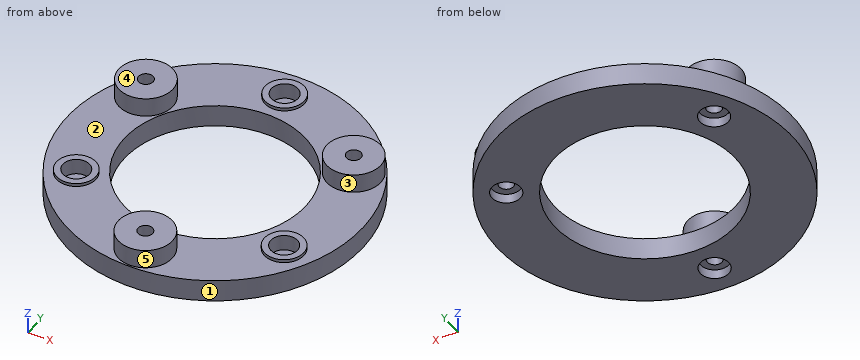
Autodesk Inventor part; units mm, degrees
ref_plane "YZ Plane" through (0, 0, 0) normal (1, 0, 0) x (0, 1, 0)
ref_plane "XZ Plane" through (0, 0, 0) normal (0, 1, 0) x (-1, 0, 0)
ref_plane "XY Plane" through (0, 0, 0) normal (0, 0, 1) x (1, 0, 0)
sketch "Skizze1" plane through (0, 0, 0) normal (0, 0, 1) x (1, 0, 0)
  line L0 (-32.55, 0) -> (32.55, 0) construction
  circle A0 centre (0, 0) radius 18.75 construction
  circle A1 centre (0, 18.75) radius 2.1
  circle A2 centre (16.238, -9.375) radius 2.1
  circle A3 centre (-16.238, -9.375) radius 2.1
  line L1 (0, 32.55) -> (0, -32.55) construction
  line L2 (0, 0) -> (-16.238, -9.375) construction
  circle A4 centre (0, 0) radius 14.25
  circle A5 centre (0, 0) radius 23.25
  circle A6 centre (0, -18.75) radius 1.15
  circle A7 centre (16.238, 9.375) radius 1.15
  circle A8 centre (-16.238, 9.375) radius 1.15
  circle A9 centre (0, -18.75) radius 4.25
  circle A10 centre (-16.238, 9.375) radius 4.25
  circle A11 centre (16.238, 9.375) radius 4.25
  circle A12 centre (0, -18.75) radius 2.25
  circle A13 centre (-16.238, 9.375) radius 2.25
  circle A14 centre (16.238, 9.375) radius 2.25
  circle A15 centre (16.238, -9.375) radius 3.1
  circle A16 centre (0, 18.75) radius 3.1
  circle A17 centre (-16.238, -9.375) radius 3.1
  dimension "d0" = 37.5
  dimension "d1" = 4.2
  dimension "d2" = 30
  dimension "d3" = 4.5
  dimension "d4" = 4.5
  dimension "d9" = 2.3
  dimension "d14" = 2
  dimension "d15" = 4.5
  dimension "d18" = 1
extrude "Extrusion2" add sketch "Skizze1" along normal blind 1.5 contours A1 | A2 | A3 | A5 | A9 | A10 | A11 | A15 | A16 | A17
extrude "Extrusion1" add sketch "Skizze1" along normal blind 2 from surface at 1.5 contours A5 | A9 | A10 | A11 | A12 | A13 | A14 | A15 | A16 | A17
extrude "Extrusion3" add sketch "Skizze1" along normal blind 3 from surface at 3.5 contours A9 | A10 | A11 | A12 | A13 | A14
extrude "Extrusion4" add sketch "Skizze1" along normal blind 0.5 from surface at 3.5 contours A15 | A16 | A17
equation "\"d3\" = d4"
properties part number "PlanetaryHolderBottom"
Work out the finished part from the listing and answer in its coordinate system (mm). Face numbers are marked on the shaded views. A direction names the side the tool comes from. Round coordinates to 2 decimals unless told otherwise and drop trailing zeros. Write each loop counter-clockwise with the first axis right and the second up, starting at its lowest first coordinate (ties: lowest second). Pieces come first, ordered by that corner, then holes. Notation, with made-up numbers: (-37, 34) - (19, 34) arc R19 ccw to (19, 63) - close; hole circle Ø4 at (87, 18). An arc over 180 degrees is marked (long way). Return JSON: item names as keys, results as strings. Group by question number.
Q1. The part is cut by section D-D on y = -10.5. Write down the section's boundary in (x, z).
Q2. The part is cut by section A-A on y = 0. Write down the section's boundary in (x, z).
Q3. Find the intervals of material crossed by L1, parallel to Y at x = 0, z = 1.2; L2, parallel to Y at x = 1.5, z = 3.75; L3, parallel to Z at x = 17.5, y = 4, in increasing order.
Q4. The mould has two halves that part along X. Classify the marked faces 3, 4 and 5: released by +X, released by -X, zero draft, split by the parting line, or undercut.
Q5. For the marked faces 1 and 2, determine the directions among +Z, -Z, +X, -X, +Y, -Y from which every point of the face is accessible in a straight line to the end or side of a thin tool.
Q6. The part is cut by section B-B on x = 0. Write down the section's boundary in (y, z).
Q7. The part is cut by section C-C on x = -10. Write down the section's boundary in (y, z).
Q8. Each of these flat-tipped pins is pushed along its axis until it touches: pin 1 Ø4.5 at (x, y) = (-0.5, 19.5) entering from +Z; pin 2 Ø4 at (x, y) = (16.238, 9.375) entering from +Z; pin 3 Ø1.3 at (x, y) = (0.5, -18.5) entering from -Z; pin 4 Ø2 at (x, y) = (16, -9) entering from +Z. Where does it stop, or does it pass through?
Solved:
{
 "1": {"outline": "(-20.74, 0) - (-9.63, 0) - (-9.63, 3.5) - (-13.35, 3.5) - (-13.35, 4) - (-14.46, 4) - (-14.46, 1.5) - (-18.01, 1.5) - (-18.01, 4) - (-19.13, 4) - (-19.13, 3.5) - (-20.74, 3.5) - close; (9.63, 0) - (20.74, 0) - (20.74, 3.5) - (19.13, 3.5) - (19.13, 4) - (18.01, 4) - (18.01, 1.5) - (14.46, 1.5) - (14.46, 4) - (13.35, 4) - (13.35, 3.5) - (9.63, 3.5) - close"},
 "2": {"outline": "(-23.25, 0) - (-14.25, 0) - (-14.25, 3.5) - (-23.25, 3.5) - close; (14.25, 0) - (23.25, 0) - (23.25, 3.5) - (14.25, 3.5) - close"},
 "3": {"L1": "-23.25 to -21, -16.5 to -14.25, 14.25 to 23.25", "L2": "-22.73 to -14.77, 16.04 to 17.28, 20.22 to 21.46", "L3": "0 to 3.5"},
 "4": {"face 3": "undercut", "face 4": "zero draft", "face 5": "split by the parting line"},
 "5": {"face 1": "+Z, -Z", "face 2": "+Z"},
 "6": {"outline": "(-23.25, 0) - (-21, 0) - (-21, 1.5) - (-19.9, 1.5) - (-19.9, 6.5) - (-23, 6.5) - (-23, 3.5) - (-23.25, 3.5) - close; (-17.6, 1.5) - (-16.5, 1.5) - (-16.5, 0) - (-14.25, 0) - (-14.25, 3.5) - (-14.5, 3.5) - (-14.5, 6.5) - (-17.6, 6.5) - close; (14.25, 0) - (23.25, 0) - (23.25, 3.5) - (21.85, 3.5) - (21.85, 4) - (20.85, 4) - (20.85, 1.5) - (16.65, 1.5) - (16.65, 4) - (15.65, 4) - (15.65, 3.5) - (14.25, 3.5) - close"},
 "7": {"outline": "(-20.99, 0) - (-10.15, 0) - (-10.15, 3.5) - (-20.99, 3.5) - close; (10.15, 0) - (20.99, 0) - (20.99, 3.5) - (10.15, 3.5) - close"},
 "8": {"pin 1": "z = 4", "pin 2": "z = 6.5", "pin 3": "z = 1.5", "pin 4": "z = 1.5"}
}
